Verification items for the finished model (mm, model axes). Face numbers are marked on the shaded views. A direction names the side the tool comes from. Coordinates: 2 decimals unless noted, no trailing zeros. Order: outer loops, then holes, each group sorted by start corner. A loop starts at its lowest first (then second) coordinate and runs counter-clockwise, first axis right, second up. Notation, with made-up numbers: M 8,10 L 47,10 A33 cw 47,42 Z; hole C 0.25,-14 d8. An arc over 180 degrees is marked long. Return JSON: item names as keys, results as strings.
```python
from build123d import *

# Parameters (mm, degrees)
PAD007_DEPTH            = 22
SKETCH025_W             = 6.8
SKETCH025_H             = 6
POCKET_DEPTH            = 21
SKETCH026_R             = 1.5
POCKET001_DEPTH         = 17.808107
POCKET002_DEPTH         = 2.5
HOLE_D                  = 3
HOLE_DEPTH              = 25
HOLE_CSINK_D            = 5
HOLE_CSINK_ANGLE        = 90
BODY007_ROLL_ANGLE      = 90
BODY007_PLACEMENT_ANGLE = 90


with BuildPart() as part:
    # Sketch024 → Pad007 (new body)
    with BuildSketch(Plane.XY):
        with BuildLine():
            Line((4.707107, 1.5), (4.707107, -17))
            ThreePointArc((1.707107, -20), (3.828427, -19.12132), (4.707107, -17))
            Line((1.707107, -20), (-10.1, -20))
            ThreePointArc((-13.1, -17), (-12.22132, -19.12132), (-10.1, -20))
            Line((-13.1, -17), (-13.1, 6))
            ThreePointArc((-12.1, 7), (-12.807107, 6.707107), (-13.1, 6))
            Line((-12.1, 7), (-11.1, 7))
            Line((-11.1, 7), (-11.1, -17))
            ThreePointArc((-11.1, -17), (-10.807107, -17.707107), (-10.1, -18))
            Line((-10.1, -18), (1.707107, -18))
            ThreePointArc((1.707107, -18), (2.414214, -17.707107), (2.707107, -17))
            Line((2.707107, -17), (2.707107, -5.207107))
            ThreePointArc((2.707107, -5.207107), (2.630986, -4.824423), (2.414214, -4.5))
            Line((2.414214, -4.5), (0.707107, -2.792893))
            ThreePointArc((0.707107, -2.792893), (0.382683, -2.57612), (0, -2.5))
            Line((0, -2.5), (-8.8, -2.5))
            Line((-8.8, -2.5), (-8.8, 0))
            Line((-8.8, 0), (-8.8, 2.5))
            Line((-8.8, 2.5), (3.707107, 2.5))
            ThreePointArc((4.707107, 1.5), (4.414214, 2.207107), (3.707107, 2.5))
        make_face()
    extrude(amount=PAD007_DEPTH)

    # Sketch025 (on Face19 of Pad007) → Pocket (cut)
    with BuildSketch(Plane(origin=(0, 0, 0), x_dir=(1, 0, 0), z_dir=(0, 0, -1))):
        with Locations((-3.4, 0)):
            Rectangle(SKETCH025_W, SKETCH025_H)
    extrude(amount=-POCKET_DEPTH, mode=Mode.SUBTRACT)

    # Sketch026 (on Face1 of Pocket) → Pocket001 (cut, through all)
    with BuildSketch(Plane.YZ.offset(4.707107)):
        with Locations((0, 14.7)):
            Circle(SKETCH026_R)
        with Locations((0, 5.2)):
            Circle(SKETCH026_R)
    extrude(amount=-POCKET001_DEPTH, mode=Mode.SUBTRACT)

    # Sketch027 (on Face21 of Pocket001) → Pocket002 (cut)
    with BuildSketch(Plane(origin=(0, 0, 0), x_dir=(0, -1, 0), z_dir=(-1, 0, 0))):
        Polygon((0, 11.640044), (2.65, 13.170022), (2.65, 16.229978), (0, 17.759956), (-2.65, 16.229978), (-2.65, 13.170022), align=None)
        Polygon((0, 8.259956), (-2.65, 6.729978), (-2.65, 3.670022), (0, 2.140044), (2.65, 3.670022), (2.65, 6.729978), align=None)
    extrude(amount=-POCKET002_DEPTH, mode=Mode.SUBTRACT)

    # Hole
    with Locations(Plane(origin=(-13.1, 0, 0), x_dir=(0, -1, 0), z_dir=(-1, 0, 0))):
        with Locations((0, 14.7), (0, 5.2)):
            CounterSinkHole(HOLE_D / 2, HOLE_CSINK_D / 2, depth=HOLE_DEPTH, counter_sink_angle=HOLE_CSINK_ANGLE)


with BuildPart() as part_1:
    # Body007 roll: moved
    add(part.part.rotate(Axis((0, 0, 0), (1, 0, 0)), BODY007_ROLL_ANGLE))


with BuildPart() as part_2:
    # Body007 placement: moved
    add(part_1.part.moved(Location((154.5, 97.2, -15.5))).rotate(Axis((154.5, 97.2, -15.5), (0, 0, 1)), BODY007_PLACEMENT_ANGLE))


solid = part_2.part
```
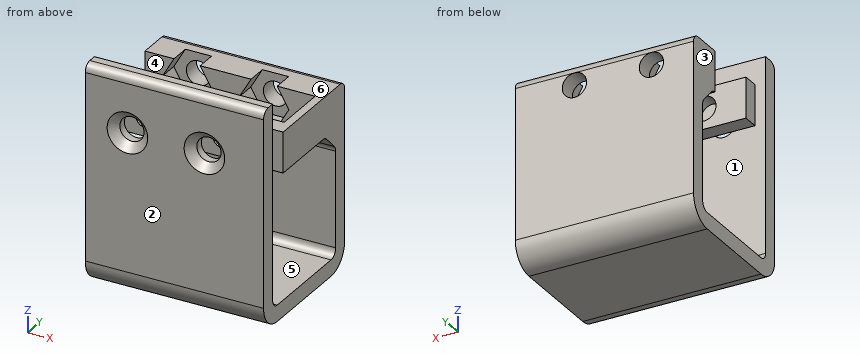
Q1. Material ranges on line 1 along X through (y, z) = (89.7, -15.5); line 2 along Y through (x, z) = (158.75, -31.5); line 3 along Z through (x, y) = (164, 89), recorded low to high.
Values:
{"line 1": "154.5 to 158.2, 161.2 to 167.7, 170.7 to 176.5", "line 2": "84.1 to 86.1, 99.91 to 101.91", "line 3": "-35.5 to -33.5, -18 to -13"}
Q2. Go/stop test with flat-tipped pins: pin 1 (4 mm diameter, centred on x = 164.5, y = 95.5, fed in from +Z); pin 2 (1.5 mm diameter, centred on y = 94.5, z = -15, fed in from -X); pin 3 (1.5 mm diameter, centred on x = 168, z = -14.5, fed in from -Y); pin 4 (5 mm diameter, centred on y = 96.5, z = -28.5, fed in from -X). Record where each tip stops, or that it passes through.
Values:
{"pin 1": "z = -13", "pin 2": "x = 175.5", "pin 3": "y = 84.29", "pin 4": "through"}
Q3. Cross-section at B-B, the plane x = 163.75. Record the boundary of the cut face in (y, z), and give its area (3 significant figures).
Values:
{"outline": "M 84.1,-32.5 A3 ccw 87.1,-35.5 L 98.91,-35.5 A3 ccw 101.91,-32.5 L 101.91,-14 A1 ccw 100.91,-13 L 97.2,-13 L 97.2,-18 A1 cw 97.91,-18.29 L 99.61,-20 A1 cw 99.91,-20.71 L 99.91,-32.5 A1 cw 98.91,-33.5 L 87.1,-33.5 A1 cw 86.1,-32.5 L 86.1,-8.5 L 85.1,-8.5 A1 ccw 84.1,-9.5 Z; M 88.4,-18 L 90.4,-18 L 90.4,-13 L 88.4,-13 Z", "area": "149 mm^2"}
Q4. Cross-section at C-C, the plane z = -25.75. Record the boundary of the cut face in (x, y), and give its area (3 significant figures).
Values:
{"outline": "M 154.5,84.1 L 176.5,84.1 L 176.5,86.1 L 154.5,86.1 Z; M 154.5,99.91 L 176.5,99.91 L 176.5,101.91 L 154.5,101.91 Z", "area": "88.0 mm^2"}
Q5. Tool access check on the marked faces 4, 5 and 6. Record the directions out of +Z, -Z, +X, -X, +Y, -Y that give a thin tool (end or side, any length) a straight path to the whole face; none if there is none.
Values:
{"face 4": "+Z, -X", "face 5": "+X, -X", "face 6": "+Z, +X, -X, +Y"}
Q6. Cross-section at D-D, the plane z = -11. Record the boundary of the cut face in (x, y), and give its area (3 significant figures).
Values:
{"outline": "M 154.5,84.1 L 176.5,84.1 L 176.5,86.1 L 154.5,86.1 Z", "area": "44.0 mm^2"}
Q7. Cross-section at A-A, the plane y = 92. Record the boundary of the cut face in (x, z), and give its area (3 significant figures).
Values:
{"outline": "M 154.5,-35.5 L 176.5,-35.5 L 176.5,-33.5 L 154.5,-33.5 Z; M 175.5,-18 L 176.5,-18 L 176.5,-13 L 175.5,-13 Z", "area": "49.0 mm^2"}
Q8. Draft check along Y on the marked faces 1, 2 and 3. Enter one of: pulls with the +Y half, pulls with the -Y half, needs draft (parallel to the pull), parting line crosses it, or undercut.
Values:
{"face 1": "undercut", "face 2": "pulls with the -Y half", "face 3": "needs draft"}
